```python
from build123d import *

# Parameters (mm, degrees)
BOSS_EXTRUDE1_DEPTH = 14
SKETCH1_3_W         = 21
SKETCH1_3_H         = 28
BOSS_EXTRUDE2_DEPTH = 28
SKETCH1_4_W         = 14
SKETCH1_4_H         = 7
BOSS_EXTRUDE3_DEPTH = 21


with BuildPart() as part:
    # Sketch1 → Boss-Extrude1 (new body)
    with BuildSketch(Plane(origin=(0, 0, 0), x_dir=(1, 0, 0), z_dir=(0, 1, 0))):
        Polygon((11, 14), (-4, 14), (-4, -14), (11, -14), (11, -7), (25, -7), (25, 7), (11, 7), align=None)
    extrude(amount=BOSS_EXTRUDE1_DEPTH)

    # Sketch1<3> → Boss-Extrude2 (add)
    with BuildSketch(Plane(origin=(0, 0, 0), x_dir=(1, 0, 0), z_dir=(0, 1, 0))):
        with Locations((-14.5, 0)):
            Rectangle(SKETCH1_3_W, SKETCH1_3_H)
    extrude(amount=BOSS_EXTRUDE2_DEPTH)

    # Sketch1<4> → Boss-Extrude3 (add)
    with BuildSketch(Plane(origin=(0, 0, 0), x_dir=(1, 0, 0), z_dir=(0, 1, 0))):
        with Locations((18, -10.5)):
            Rectangle(SKETCH1_4_W, SKETCH1_4_H)
        with Locations((18, 10.5)):
            Rectangle(SKETCH1_4_W, SKETCH1_4_H)
    extrude(amount=BOSS_EXTRUDE3_DEPTH)


solid = part.part
```
Part model, mm, in its own coordinate system. A direction names the side the tool comes from. Coordinates: 2 decimals unless noted, no trailing zeros. Order: outer loops, then holes, each group sorted by start corner. A loop starts at its lowest first (then second) coordinate and runs counter-clockwise, first axis right, second up. Notation, with made-up numbers: (-36, 68) -> (-28, 68) arc R20 cw to (-28, 103) -> close; hole circle Ø2 at (39.5, 22). An arc over 180 degrees is marked (long way). Put each result on its own line as item: value. Start each with the question number.
(1) Which spindle directions (+Z, -Z, +X, -X, +Y, -Y) get a long thin tool onto all of the face, cutting with end or side? Do faces 5 (the face through (18, 17, -7)), 6 (the face through (18, 21, -11)), 7 (the face through (11, 17, -10)), 8 (the face through (-15, 28, 0)). Say none if no direction does.
(2) Band-saw the part on A-A (y = 18.75). Give the cut face in (x, z), then the cut area to 3 significant figures.
(3) Mould opens along X. For faces 1 (the face through (25, 8, 0)), 2 (the face through (18, 21, 10)), 3 (the face through (11, 17, 11)), 4 (the face through (-4, 21, 0)) say: pulls with the +X half, pulls with the -X half, needs draft (parallel to the pull), parting line crosses it, or undercut.
(4) Band-saw the part on D-D (z = 10.5). Give the cut face in (x, y), then the cut area to 3 significant figures.
(5) Band-saw the part on B-B (z = 2.75). Give the cut face in (x, y), then the cut area to 3 significant figures.
(6) Band-saw the part on C-C (x = 18). Give the cut face in (y, z).
(7) Pin check, flat tip, straight feed: pin 1 Ø14 at (x, z) = (10.5, -2) entering from +Y. Stop position of the tip, or through.
(8) Probe line 1 along X through (y, z) = (18.75, 11.75); line 2 along Y through (x, z) = (0, -5); line 3 along Y through (x, z) = (20.5, 9.5). List the from-to ranges inside material, lowest first. Write a range as [from, to].
Determined:
1. face 5: +X, +Y
1. face 6: +Z, -Z, +X, +Y
1. face 7: +Z, -Z, +Y
1. face 8: +Z, -Z, +X, -X, +Y
2. outline: (-25, -14) -> (-4, -14) -> (-4, 14) -> (-25, 14) -> close; (11, -14) -> (25, -14) -> (25, -7) -> (11, -7) -> close; (11, 7) -> (25, 7) -> (25, 14) -> (11, 14) -> close
2. area: 784 mm²
3. face 1: pulls with the +X half
3. face 2: needs draft
3. face 3: undercut
3. face 4: undercut
4. outline: (-25, 0) -> (25, 0) -> (25, 21) -> (11, 21) -> (11, 14) -> (-4, 14) -> (-4, 28) -> (-25, 28) -> close
4. area: 1,090 mm²
5. outline: (-25, 0) -> (25, 0) -> (25, 14) -> (-4, 14) -> (-4, 28) -> (-25, 28) -> close
5. area: 994 mm²
6. outline: (0, -14) -> (21, -14) -> (21, -7) -> (14, -7) -> (14, 7) -> (21, 7) -> (21, 14) -> (0, 14) -> close
7. pin 1: stops at y = 21
8. line 1: x = [-25, -4], [11, 25]
8. line 2: y = [0, 14]
8. line 3: y = [0, 21]
